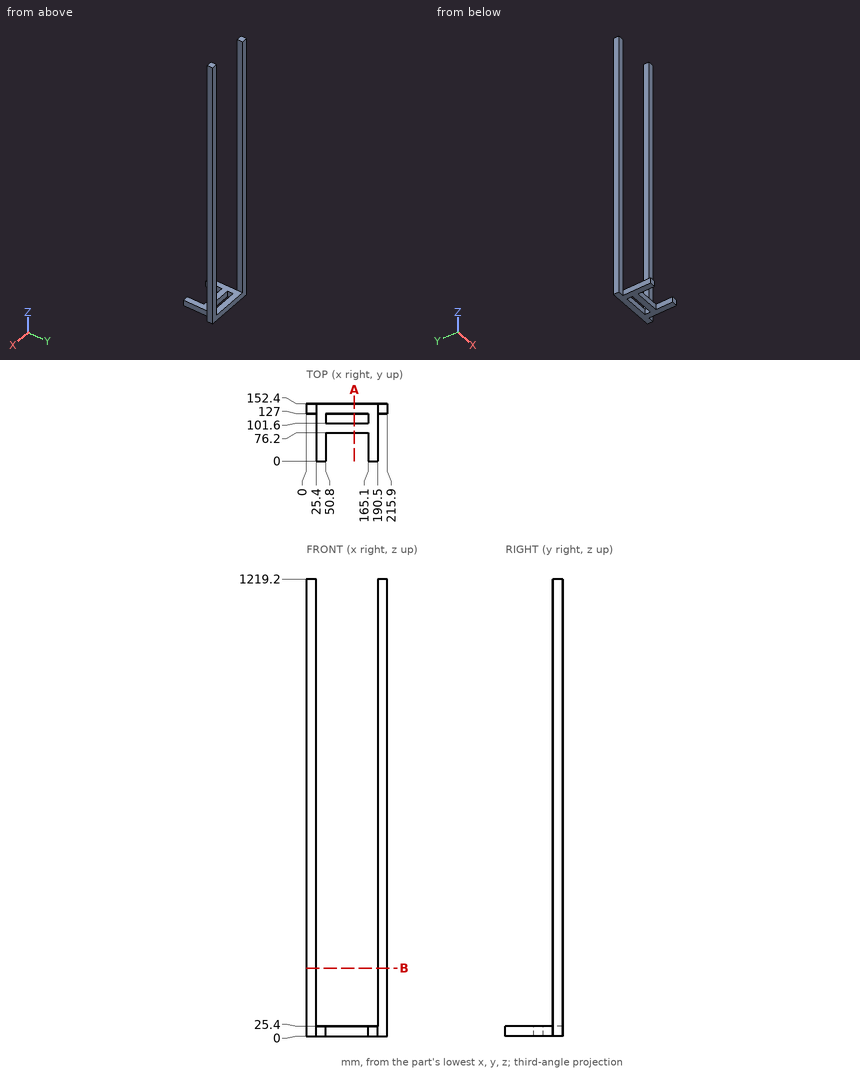
Geometry check sheet. Reference: drawing and pictorial views, mm from the part's lowest x, y, z. Round coordinates to 2 decimals unless told otherwise and drop trailing zeros. Order: outer loops, then holes, each group sorted by start corner. A loop starts at its lowest first (then second) coordinate and runs counter-clockwise, first axis right, second up.
Q1. Depth check by flat-ended pin: P1, Ø7.5, axis at x = 203, z = 838, coming from the -Y side; P2, Ø20.5, axis at y = 45.5, z = 7.5, coming from the +X side; P3, Ø7.5, axis at y = 117.5, z = 13.5, coming from the -X side. Enter the tip coordinate at first touch or a pass-through.
Filled sheet:
P1: stops at y = 127
P2: stops at x = 190.5
P3: stops at x = 25.4
Q2. Cross-section at A-A, the plane x = 128. Enter the section's corners in (y, z).
Filled sheet:
outline: (76.2, 0) - (101.6, 0) - (101.6, 25.4) - (76.2, 25.4) - close; (127, 0) - (152.4, 0) - (152.4, 25.4) - (127, 25.4) - close
Q3. Scan lines: L1, parallel to X at y = 145, z = 896; L2, parallel to Z at x = 27, y = 52.5; L3, parallel to Y at x = 200.5, z = 496. Record each from-to range of solid material in increasing order.
Filled sheet:
L1: x = 0 to 25.4, 190.5 to 215.9
L2: z = 0 to 25.4
L3: y = 127 to 152.4
Q4. Cross-section at B-B, the plane z = 181. Enter the section's corners in (x, y), plus the area to 3 significant figures.
Filled sheet:
outline: (0, 127) - (25.4, 127) - (25.4, 152.4) - (0, 152.4) - close; (190.5, 127) - (215.9, 127) - (215.9, 152.4) - (190.5, 152.4) - close
area: 1,290 mm2
